from build123d import *

# Parameters (mm, degrees)
SKETCH1_R           = 32
BOSS_EXTRUDE1_DEPTH = 13.5
FILLET1_R           = 1
FILLET2_R           = 1
SKETCH2_R           = 2.5
BOSS_EXTRUDE2_DEPTH = 50


with BuildPart() as part:
    # Sketch1 → Boss-Extrude1 (new, symmetric)
    with BuildSketch(Plane(origin=(0, 0, 0), x_dir=(1, 0, 0), z_dir=(0, 1, 0))):
        with Locations(Location((0, 0, 0), (0, 0, 270))):
            Circle(SKETCH1_R)
    extrude(amount=BOSS_EXTRUDE1_DEPTH, both=True)

    # Fillet1
    fillet1_edges = [part.edges().sort_by_distance(p)[0] for p in [
        (0, -13.5, -32),
    ]]
    fillet(fillet1_edges, radius=FILLET1_R)

    # Fillet2
    fillet2_edges = [part.edges().sort_by_distance(p)[0] for p in [
        (0, 13.5, -32),
    ]]
    fillet(fillet2_edges, radius=FILLET2_R)

    # Sketch2 → Boss-Extrude2 (add)
    with BuildSketch(Plane(origin=(0, -13.5, 0), x_dir=(-1, 0, 0), z_dir=(0, -1, 0))):
        with Locations(Location((0, 0, 0), (0, 0, 270))):
            Circle(SKETCH2_R)
    extrude(amount=BOSS_EXTRUDE2_DEPTH)


solid = part.part
Source: CAD feature listing. Evaluate the final solid. Frame: model axes, mm. A direction names the side the tool comes from. Round coordinates to 2 decimals unless told otherwise and drop trailing zeros. Write each loop counter-clockwise with the first axis right and the second up, starting at its lowest first coordinate (ties: lowest second). Pieces come first, ordered by that corner, then holes. Notation, with made-up numbers: (-32, -13.75) - (-12, -13.75) arc R25 ccw to (-12, 14.25) - close; hole circle Ø5 at (-17, 62.5). An arc over 180 degrees is marked (long way). Use CSV: the item, a comma, the result in double quotes. Start each with the question number.
(1) Cut plane D-D, the plane y = 0. Return loops of the section in (x, z), and give its area (3 significant figures).
(2) Set-up query: faces 1 (the face through (0, 13.5, 0)), 2 (the face through (2.44, -38.15, -0.54)). Return all of +Z, -Z, +X, -X, +Y, -Y with unobstructed straight access to the full face (end or side cutting, diameter ignored); none if empty.
(3) Material intervals for probe 1 along Y at (x, z) = (-25, -6.5); probe 2 along Z at (x, y) = (-1, -8.5); probe 3 along X at (y, z) = (-6.5, -23), sorted ascending. Write a range as [from, to].
(4) First-contact query: pin 1 Ø12 at (x, y) = (-14, -54) entering from -Z; pin 2 Ø4 at (y, z) = (4.5, -6) entering from -X; pin 3 Ø2 at (x, z) = (22.5, -16) entering from -Y; pin 4 Ø12 at (x, y) = (14, 3.5) entering from +Z. Flat tips, straight axial feed; report the tip coordinate or a pass-through.
(5) Cut plane B-B, the plane z = 0. Return loops of the section in (x, y).
(6) Cut plane C-C, the plane y = -31. Return loops of the section in (x, z).
(7) Cut plane A-A, the plane x = 0. Return loops of the section in (y, z).
Geometry says:
1,outline,"circle Ø64 at (0, 0)"
1,area,"3,220 mm²"
2,face 1,"+Z, -Z, +X, -X, +Y"
2,face 2,"-Y"
3,probe 1,"[-13.5, 13.5]"
3,probe 2,"[-31.98, 31.98]"
3,probe 3,"[-22.25, 22.25]"
4,pin 1,"through"
4,pin 2,"x = -31.75"
4,pin 3,"y = -13.5"
4,pin 4,"z = 30.98"
5,outline,"(-32, -12.5) arc R1 ccw to (-31, -13.5) - (-2.5, -13.5) - (-2.5, -63.5) - (2.5, -63.5) - (2.5, -13.5) - (31, -13.5) arc R1 ccw to (32, -12.5) - (32, 12.5) arc R1 ccw to (31, 13.5) - (-31, 13.5) arc R1 ccw to (-32, 12.5) - close"
6,outline,"circle Ø5 at (0, 0)"
7,outline,"(-63.5, -2.5) - (-13.5, -2.5) - (-13.5, -31) arc R1 ccw to (-12.5, -32) - (12.5, -32) arc R1 ccw to (13.5, -31) - (13.5, 31) arc R1 ccw to (12.5, 32) - (-12.5, 32) arc R1 ccw to (-13.5, 31) - (-13.5, 2.5) - (-63.5, 2.5) - close"
